Geometry check sheet. Reference: the model listing, model coordinates, mm. A direction names the side the tool comes from. Give positions to 0.01 mm unless a question says otherwise; leave off trailing zeros. Write each loop counter-clockwise with the first axis right and the second up, starting at its lowest first coordinate (ties: lowest second). Pieces come first, ordered by that corner, then holes. Notation, with made-up numbers: (-38.5, 21) - (8.5, 21) arc R11 cw to (8.5, 33) - close; hole circle Ø11 at (71, -19.75). An arc over 180 degrees is marked (long way). Use a Markdown table: item, result.
```python
from build123d import *

# Parameters (mm, degrees)
SKETCH2_W                       = 122
SKETCH2_H                       = 82
BOSS_EXTRUDE1_DEPTH             = 5
SKETCH2_3_W                     = 122
SKETCH2_3_H                     = 82
BOSS_EXTRUDE2_DEPTH             = 10
F_0_80_TAPPED_HOLE1_D           = 1.19126
F_0_80_TAPPED_HOLE1_DEPTH       = 3.642109389
F_0_80_TAPPED_HOLE1_CSINK_D     = 2.794
F_0_80_TAPPED_HOLE1_CSINK_ANGLE = 90
F_0_80_TAPPED_HOLE1_TIP         = 0.357890611
SKETCH8_W                       = 38
SKETCH8_H                       = 5
CUT_EXTRUDE1_DEPTH              = 5
CUT_EXTRUDE2_DEPTH              = 5
CUT_EXTRUDE3_DEPTH              = 5


with BuildPart() as part:
    # Sketch2 → Boss-Extrude1 (new body)
    # profile 1 of 2: a face of its own
    with BuildSketch(Plane(origin=(0, 0, 0), x_dir=(1, 0, 0), z_dir=(0, 1, 0))):
        with BuildLine():
            ThreePointArc((-66, 41), (-64.535533906, 44.535533906), (-61, 46))
            Line((-61, 46), (61, 46))
            ThreePointArc((61, 46), (64.535533906, 44.535533906), (66, 41))
            Line((66, 41), (66, -41))
            ThreePointArc((66, -41), (64.535533906, -44.535533906), (61, -46))
            Line((61, -46), (-61, -46))
            ThreePointArc((-61, -46), (-64.535533906, -44.535533906), (-66, -41))
            Line((-66, -41), (-66, 41))
        make_face()
        Rectangle(SKETCH2_W, SKETCH2_H, mode=Mode.SUBTRACT)
    # profile 2 of 2: a face of its own
    with BuildSketch(Plane(origin=(0, 0, 0), x_dir=(1, 0, 0), z_dir=(0, 1, 0))):
        Rectangle(SKETCH2_W, SKETCH2_H)
    extrude(amount=BOSS_EXTRUDE1_DEPTH)

    # Sketch2<3> → Boss-Extrude2 (add)
    with BuildSketch(Plane(origin=(0, 0, 0), x_dir=(1, 0, 0), z_dir=(0, 1, 0))):
        with BuildLine():
            Line((-61, -46), (61, -46))
            ThreePointArc((61, -46), (64.535533906, -44.535533906), (66, -41))
            Line((66, -41), (66, 41))
            ThreePointArc((66, 41), (64.535533906, 44.535533906), (61, 46))
            Line((61, 46), (-61, 46))
            ThreePointArc((-61, 46), (-64.535533906, 44.535533906), (-66, 41))
            Line((-66, 41), (-66, -41))
            ThreePointArc((-66, -41), (-64.535533906, -44.535533906), (-61, -46))
        make_face()
        Rectangle(SKETCH2_3_W, SKETCH2_3_H, mode=Mode.SUBTRACT)
    extrude(amount=BOSS_EXTRUDE2_DEPTH)

    # #0-80 Tapped Hole1
    with Locations(Plane(origin=(62.880041054, 10, -42.889125675), x_dir=(0, 0, 1), z_dir=(0, 1, 0))):
        with Locations((0, 0), (85.769428086, 0), (0, -125.638471979), (85.769428086, -125.638471979)):
            CounterSinkHole(F_0_80_TAPPED_HOLE1_D / 2, F_0_80_TAPPED_HOLE1_CSINK_D / 2, depth=F_0_80_TAPPED_HOLE1_DEPTH, counter_sink_angle=F_0_80_TAPPED_HOLE1_CSINK_ANGLE)
            with Locations((0, 0, -(F_0_80_TAPPED_HOLE1_DEPTH + F_0_80_TAPPED_HOLE1_TIP / 2))):  # 118° drill point
                Cone(0, F_0_80_TAPPED_HOLE1_D / 2, F_0_80_TAPPED_HOLE1_TIP, mode=Mode.SUBTRACT)

    # Sketch8 → Cut-Extrude1 (cut)
    with BuildSketch(Plane(origin=(0, 10, 0), x_dir=(1, 0, 0), z_dir=(0, 1, 0))):
        with Locations((-26, 43.5)):
            Rectangle(SKETCH8_W, SKETCH8_H)
    extrude(amount=-CUT_EXTRUDE1_DEPTH, mode=Mode.SUBTRACT)

    # Sketch9 → Cut-Extrude2 (cut)
    with BuildSketch(Plane(origin=(0, 0, -46), x_dir=(-1, 0, 0), z_dir=(0, 0, -1))):
        with BuildLine():
            Line((-20.5, 10), (-20.5, 8))
            ThreePointArc((-20.5, 8), (-17.5, 5), (-14.5, 8))
            Line((-14.5, 8), (-14.5, 10))
            Line((-14.5, 10), (-20.5, 10))
        make_face()
    extrude(amount=-CUT_EXTRUDE2_DEPTH, mode=Mode.SUBTRACT)

    # Sketch10 → Cut-Extrude3 (cut)
    with BuildSketch(Plane(origin=(0, 0, -46), x_dir=(-1, 0, 0), z_dir=(0, 0, -1))):
        with BuildLine():
            Line((52.5, 10), (52.5, 8))
            ThreePointArc((52.5, 8), (55.5, 5), (58.5, 8))
            Line((58.5, 8), (58.5, 10))
            Line((58.5, 10), (52.5, 10))
        make_face()
    extrude(amount=-CUT_EXTRUDE3_DEPTH, mode=Mode.SUBTRACT)


solid = part.part
```
1) Section check B-B on x = 7. Record the boundary of the cut face in (y, z), then the cut area to 3 significant figures.
Working result:
| item | result |
|---|---|
| outline | (0, -46) - (10, -46) - (10, -41) - (5, -41) - (5, 41) - (10, 41) - (10, 46) - (0, 46) - close |
| area | 510 mm² |
2) Material ranges on L1, parallel to Z at x = 35, y = 7; L2, parallel to X at y = 7, z = -26.5; L3, parallel to Y at x = -47.5, z = 32, recorded low to high. Write a range as from..to.
Working result:
| item | result |
|---|---|
| L1 | z = -46..-41, 41..46 |
| L2 | x = -66..-61, 61..66 |
| L3 | y = 0..5 |
3) Section check C-C on x = -25. Record the boundary of the cut face in (y, z).
Working result:
| item | result |
|---|---|
| outline | (0, -46) - (5, -46) - (5, 41) - (10, 41) - (10, 46) - (0, 46) - close |
4) Set-up check for faces 1 (the flat face through (-60, 7, -41)), 2 (the flat face through (1, 5, 46)), 3 (the flat face through (-7, 8, -43)): record each of +Z, -Z, +X, -X, +Y, -Y from which the full face is reachable in a straight line by a thin tool's end or side.
Working result:
| item | result |
|---|---|
| face 1 | +Y |
| face 2 | +Z, +X, -X, +Y, -Y |
| face 3 | -Z, +Y |
5) Section check A-A on z = -16. Record the boundary of the cut face in (x, y).
Working result:
| item | result |
|---|---|
| outline | (-66, 0) - (66, 0) - (66, 10) - (61, 10) - (61, 5) - (-61, 5) - (-61, 10) - (-66, 10) - close |
6) Depth check by flat-ended pin: P1, Ø4, axis at x = 16.5, z = -20.5, coming from the -Y side; P2, Ø1.6, axis at y = 9.5, z = -43, coming from the -X side; P3, Ø2, axis at y = 9.5, z = -44.5, coming from the +X side; P4, Ø5, axis at x = 13.5, z = 12.5, coming from the +Y side. Enter the tip coordinate at first touch or a pass-through.
Working result:
| item | result |
|---|---|
| P1 | stops at y = 0 |
| P2 | stops at x = -65.85 |
| P3 | stops at x = 65.33 |
| P4 | stops at y = 5 |
7) Mould release check, pull along Z, two halves, no side actions. Record for faces 4 (the flat face through (-66, 5, 1)), 5 (the flat face through (-61, 7, 1)), 6 (the cylindrical face through (65, 5, 44)), 7 (the flat face through (13, 4, -46)): pulls with the +Z half, pulls with the -Z half, needs draft (parallel to the pull), parting line crosses it, or undercut.
Working result:
| item | result |
|---|---|
| face 4 | needs draft |
| face 5 | undercut |
| face 6 | pulls with the +Z half |
| face 7 | pulls with the -Z half |
